For this review, take the finished solid that the model builds, in its own axes (mm). A direction names the side the tool comes from. Give positions to 0.01 mm unless a question says otherwise; leave off trailing zeros. Loops run counter-clockwise (first coordinate to the right, second up) from the corner with the lowest first, then second, coordinate; pieces in that order, holes last. Notation, with made-up numbers: (58.25, -33) - (71.25, -33) arc R19 cw to (71.25, -6) - close; hole circle Ø7 at (-23, 50.25). An arc over 180 degrees is marked (long way). Answer as CSV lines item,"result".
from build123d import *

# Parameters (mm, degrees)
F0_W     = 38.1
F0_H     = 42.037
F1_DEPTH = 15.875
F2_R     = 3.175
F3_DEPTH = 15.876
F4_R     = 14.097
F5_DEPTH = 12.7
F6_R     = 1.397
F6_R_2   = 1.778
F7_DEPTH = 3.176
F8_R     = 1.5875
F9_DEPTH = 42.038


with BuildPart() as f1:
    # F0 (on Front) → F1 (new body)
    with BuildSketch(Plane.XZ):
        Rectangle(F0_W, F0_H)
    extrude(amount=F1_DEPTH)

    # F2 (on face) → F3 (cut, through all)
    with BuildSketch(Plane.XZ.offset(15.875)):
        Circle(F2_R)
    extrude(amount=-F3_DEPTH, mode=Mode.SUBTRACT)

    # F4 (on face) → F5 (cut)
    with BuildSketch(Plane.XZ.offset(15.875)):
        Circle(F4_R)
    extrude(amount=-F5_DEPTH, mode=Mode.SUBTRACT)

    # F6 (on face) → F7 (cut, through all)
    with BuildSketch(Plane.XZ.offset(3.175)):
        with Locations((0, 7.874)):
            Circle(F6_R)
        with Locations((-9.3472, 0)):
            Circle(F6_R_2)
        with Locations((0, -7.874)):
            Circle(F6_R)
        with Locations((9.3472, 0)):
            Circle(F6_R_2)
    extrude(amount=-F7_DEPTH, mode=Mode.SUBTRACT)

    # F8 (on face) → F9 (cut, through all)
    with BuildSketch(Plane(origin=(0, 0, -21.0185), x_dir=(1, 0, 0), z_dir=(0, 0, -1))):
        with Locations((-14.351, 7.9502)):
            Circle(F8_R)
        with Locations((14.351, 7.9375)):
            Circle(F8_R)
    extrude(amount=-F9_DEPTH, mode=Mode.SUBTRACT)


solid = f1.part
1) Consider section C-C on z = 0. Count the separate pieces of the cut face and the enclosed holes in it, and give its area (3 significant figures).
From the geometry:
separate pieces,"4"
enclosed holes,"0"
area,"195 mm^2"
2) Machinability: for faces 5 (the cylindrical face through (-0.69, -1.61, -3.1)), 6 (the cylindrical face through (-11.187, -9.614, -8.578)), which of the approach directions +Z, -Z, +X, -X, +Y, -Y give a long, thin tool a straight path to every point of the face, cutting with its end or side? Answer none if there is none.
From the geometry:
face 5,"+Y, -Y"
face 6,"-Y"
3) Consider section B-B on x = -15. Write out the cut boundary in (y, z) (1 decimal).
From the geometry:
outline,"(-15.9, -21) - (-9.4, -21) - (-9.4, 21) - (-15.9, 21) - close; (-6.5, -21) - (0, -21) - (0, 21) - (-6.5, 21) - close"
4) Wall thickness on line 1 (X direction, y = -6.75, z = -10.5); line 2 (X direction, y = -9.25, z = -7); line 3 (Z direction, x = 6.5, y = -7.5): over which ranges is each line inside the solid? List them lowest first. Write a range as from..to.
From the geometry:
line 1,"x = -19.05..-15.39, -13.31..-9.41, 9.41..13.3, 15.4..19.05"
line 2,"x = -19.05..-15.26, -13.44..-12.24, 12.24..13.46, 15.24..19.05"
line 3,"z = -21.02..-12.51, 12.51..21.02"
5) Consider section A-A on x = 0. Write out the cut boundary in (y, z) (1 decimal).
From the geometry:
outline,"(-15.9, -21) - (0, -21) - (0, -9.3) - (-3.2, -9.3) - (-3.2, -14.1) - (-15.9, -14.1) - close; (-15.9, 14.1) - (-3.2, 14.1) - (-3.2, 9.3) - (0, 9.3) - (0, 21) - (-15.9, 21) - close; (-3.2, -6.5) - (0, -6.5) - (0, -3.2) - (-3.2, -3.2) - close; (-3.2, 3.2) - (0, 3.2) - (0, 6.5) - (-3.2, 6.5) - close"
6) Insertion check: P1, Ø3.5, axis at x = 0, z = 7.874, coming from the -Y side (3 decimals). The pin has a flat end and moves straight along its axis. Give the tip position at first contact, or say it passes through.
From the geometry:
P1,"stops at y = -3.175"
7) Draft analysis for pull direction Z (two halves, no side actions). For faces 1 (the flat face through (0, -8, -21.018)), 2 (the cylindrical face through (15.865, -8.414, -0.294)), 3 (the flat face through (-0.2, -3.175, 3.33)), 4 (the cylindrical face through (-0.18, -1.61, 9.26)), state which applies: pulls with the +Z half, pulls with the -Z half, needs draft (parallel to the pull), parting line crosses it, or undercut.
From the geometry:
face 1,"pulls with the -Z half"
face 2,"needs draft"
face 3,"undercut"
face 4,"undercut"
